The model under review builds one solid part; all positions refer to its coordinate system, in mm. Face numbers are marked on the shaded views. Round coordinates to 2 decimals unless told otherwise and drop trailing zeros. Write each loop counter-clockwise with the first axis right and the second up, starting at its lowest first coordinate (ties: lowest second). Pieces come first, ordered by that corner, then holes. Notation, with made-up numbers: (-10, 35) - (14, 35) arc R22 cw to (14, 52) - close; hole circle Ø5 at (49.25, 73.25). An arc over 180 degrees is marked (long way). One line per question, with ' | ' between items. Start each with the question number.
```python
from build123d import *

# Parameters (mm, degrees)
BOX202_W          = 16
BOX202_H          = 6
BOX202_DEPTH      = 2
BOX208_W          = 16
BOX208_H          = 6
BOX208_DEPTH      = 2
BOX206_W          = 16
BOX206_H          = 6
BOX206_DEPTH      = 2
BOX204_W          = 16
BOX204_H          = 6
BOX204_DEPTH      = 2
BOX198_W          = 16
BOX198_H          = 6
BOX198_DEPTH      = 2
BOX209_W          = 16
BOX209_H          = 6
BOX209_DEPTH      = 2
BOX205_W          = 16
BOX205_H          = 6
BOX205_DEPTH      = 2
BOX207_W          = 16
BOX207_H          = 6
BOX207_DEPTH      = 2
BOX200_W          = 16
BOX200_H          = 6
BOX200_DEPTH      = 2
BOX212_W          = 16
BOX212_H          = 6
BOX212_DEPTH      = 2
BOX211_W          = 16
BOX211_H          = 6
BOX211_DEPTH      = 2
BOX203_W          = 16
BOX203_H          = 6
BOX203_DEPTH      = 2
CYLINDER480_R     = 1.5
CYLINDER480_DEPTH = 50
CYLINDER467_R     = 1.5
CYLINDER467_DEPTH = 50
CYLINDER483_R     = 1.5
CYLINDER483_DEPTH = 50
CYLINDER486_R     = 1.5
CYLINDER486_DEPTH = 50
CYLINDER488_R     = 1.5
CYLINDER488_DEPTH = 50
CYLINDER482_R     = 1.5
CYLINDER482_DEPTH = 50
CYLINDER476_R     = 5
CYLINDER476_DEPTH = 100
CYLINDER475_R     = 5
CYLINDER475_DEPTH = 100
CYLINDER461_R     = 5
CYLINDER461_DEPTH = 100
CYLINDER477_R     = 5
CYLINDER477_DEPTH = 100
CYLINDER481_R     = 5
CYLINDER481_DEPTH = 100
CYLINDER478_R     = 5
CYLINDER478_DEPTH = 100
CYLINDER479_R     = 5
CYLINDER479_DEPTH = 100
CYLINDER474_R     = 5
CYLINDER474_DEPTH = 100
BOX201_W          = 10
BOX201_H          = 108
BOX201_DEPTH      = 20


with BuildPart() as krychle202:
    # Box202 → Box202 (new body)
    with BuildSketch(Plane(origin=(60, 2, 16), x_dir=(1, 0, 0), z_dir=(0, 0, 1))):
        with Locations((8, 3)):
            Rectangle(BOX202_W, BOX202_H)
    extrude(amount=BOX202_DEPTH)


with BuildPart() as krychle208:
    # Box208 → Box208 (new body)
    with BuildSketch(Plane(origin=(60, -21, 10), x_dir=(1, 0, 0), z_dir=(0, 0, 1))):
        with Locations((8, 3)):
            Rectangle(BOX208_W, BOX208_H)
    extrude(amount=BOX208_DEPTH)


with BuildPart() as krychle206:
    # Box206 → Box206 (new body)
    with BuildSketch(Plane(origin=(60, -21, 16), x_dir=(1, 0, 0), z_dir=(0, 0, 1))):
        with Locations((8, 3)):
            Rectangle(BOX206_W, BOX206_H)
    extrude(amount=BOX206_DEPTH)


with BuildPart() as krychle204:
    # Box204 → Box204 (new body)
    with BuildSketch(Plane(origin=(60, -41, 10), x_dir=(1, 0, 0), z_dir=(0, 0, 1))):
        with Locations((8, 3)):
            Rectangle(BOX204_W, BOX204_H)
    extrude(amount=BOX204_DEPTH)


with BuildPart() as krychle198:
    # Box198 → Box198 (new body)
    with BuildSketch(Plane(origin=(60, -41, 16), x_dir=(1, 0, 0), z_dir=(0, 0, 1))):
        with Locations((8, 3)):
            Rectangle(BOX198_W, BOX198_H)
    extrude(amount=BOX198_DEPTH)


with BuildPart() as krychle209:
    # Box209 → Box209 (new body)
    with BuildSketch(Plane(origin=(60, -51, 10), x_dir=(1, 0, 0), z_dir=(0, 0, 1))):
        with Locations((8, 3)):
            Rectangle(BOX209_W, BOX209_H)
    extrude(amount=BOX209_DEPTH)


with BuildPart() as krychle205:
    # Box205 → Box205 (new body)
    with BuildSketch(Plane(origin=(60, -51, 16), x_dir=(1, 0, 0), z_dir=(0, 0, 1))):
        with Locations((8, 3)):
            Rectangle(BOX205_W, BOX205_H)
    extrude(amount=BOX205_DEPTH)


with BuildPart() as krychle207:
    # Box207 → Box207 (new body)
    with BuildSketch(Plane(origin=(60, 30, 10), x_dir=(1, 0, 0), z_dir=(0, 0, 1))):
        with Locations((8, 3)):
            Rectangle(BOX207_W, BOX207_H)
    extrude(amount=BOX207_DEPTH)


with BuildPart() as krychle200:
    # Box200 → Box200 (new body)
    with BuildSketch(Plane(origin=(60, 46, 10), x_dir=(1, 0, 0), z_dir=(0, 0, 1))):
        with Locations((8, 3)):
            Rectangle(BOX200_W, BOX200_H)
    extrude(amount=BOX200_DEPTH)


with BuildPart() as krychle212:
    # Box212 → Box212 (new body)
    with BuildSketch(Plane(origin=(60, 30, 16), x_dir=(1, 0, 0), z_dir=(0, 0, 1))):
        with Locations((8, 3)):
            Rectangle(BOX212_W, BOX212_H)
    extrude(amount=BOX212_DEPTH)


with BuildPart() as krychle211:
    # Box211 → Box211 (new body)
    with BuildSketch(Plane(origin=(60, 46, 16), x_dir=(1, 0, 0), z_dir=(0, 0, 1))):
        with Locations((8, 3)):
            Rectangle(BOX211_W, BOX211_H)
    extrude(amount=BOX211_DEPTH)


with BuildPart() as compound592:
    # Box203 → Box203 (new body)
    with BuildSketch(Plane(origin=(60, 2, 10), x_dir=(1, 0, 0), z_dir=(0, 0, 1))):
        with Locations((8, 3)):
            Rectangle(BOX203_W, BOX203_H)
    extrude(amount=BOX203_DEPTH)

    # Compound592: union Krychle202, Krychle208, Krychle206, Krychle204, Krychle198, Krychle209, Krychle205, Krychle207, Krychle200, Krychle212, Krychle211
    add(krychle202.part)
    add(krychle208.part)
    add(krychle206.part)
    add(krychle204.part)
    add(krychle198.part)
    add(krychle209.part)
    add(krychle205.part)
    add(krychle207.part)
    add(krychle200.part)
    add(krychle212.part)
    add(krychle211.part)


with BuildPart() as compound592_1:
    # Compound592 placement: moved
    add(compound592.part.moved(Location((39, 24, 3))))


with BuildPart() as obj1:
    # Cylinder480 → Cylinder480 (new body)
    with BuildSketch(Plane(origin=(63, -18, -12), x_dir=(1, 0, 0), z_dir=(0, 0, 1))):
        Circle(CYLINDER480_R)
    extrude(amount=CYLINDER480_DEPTH)


with BuildPart() as obj2:
    # Cylinder467 → Cylinder467 (new body)
    with BuildSketch(Plane(origin=(63, -38, -12), x_dir=(1, 0, 0), z_dir=(0, 0, 1))):
        Circle(CYLINDER467_R)
    extrude(amount=CYLINDER467_DEPTH)


with BuildPart() as obj3:
    # Cylinder483 → Cylinder483 (new body)
    with BuildSketch(Plane(origin=(63, -48, -12), x_dir=(1, 0, 0), z_dir=(0, 0, 1))):
        Circle(CYLINDER483_R)
    extrude(amount=CYLINDER483_DEPTH)


with BuildPart() as obj4:
    # Cylinder486 → Cylinder486 (new body)
    with BuildSketch(Plane(origin=(63, 33, -12), x_dir=(1, 0, 0), z_dir=(0, 0, 1))):
        Circle(CYLINDER486_R)
    extrude(amount=CYLINDER486_DEPTH)


with BuildPart() as obj5:
    # Cylinder488 → Cylinder488 (new body)
    with BuildSketch(Plane(origin=(63, 49, -12), x_dir=(1, 0, 0), z_dir=(0, 0, 1))):
        Circle(CYLINDER488_R)
    extrude(amount=CYLINDER488_DEPTH)


with BuildPart() as compound593:
    # Cylinder482 → Cylinder482 (new body)
    with BuildSketch(Plane(origin=(63, 5, -12), x_dir=(1, 0, 0), z_dir=(0, 0, 1))):
        Circle(CYLINDER482_R)
    extrude(amount=CYLINDER482_DEPTH)

    # Compound593: union obj1, obj2, obj3, obj4, obj5
    add(obj1.part)
    add(obj2.part)
    add(obj3.part)
    add(obj4.part)
    add(obj5.part)


with BuildPart() as compound593_1:
    # Compound593 placement: moved
    add(compound593.part.moved(Location((39, 24, 0))))


with BuildPart() as obj6:
    # Cylinder476 → Cylinder476 (new body)
    with BuildSketch(Plane(origin=(24, -51, 25), x_dir=(0, 0, -1), z_dir=(1, 0, 0))):
        Circle(CYLINDER476_R)
    extrude(amount=CYLINDER476_DEPTH)


with BuildPart() as obj7:
    # Cylinder475 → Cylinder475 (new body)
    with BuildSketch(Plane(origin=(24, 36, 34), x_dir=(0, 0, -1), z_dir=(1, 0, 0))):
        Circle(CYLINDER475_R)
    extrude(amount=CYLINDER475_DEPTH)


with BuildPart() as obj8:
    # Cylinder461 → Cylinder461 (new body)
    with BuildSketch(Plane(origin=(24, -36, 34), x_dir=(0, 0, -1), z_dir=(1, 0, 0))):
        Circle(CYLINDER461_R)
    extrude(amount=CYLINDER461_DEPTH)


with BuildPart() as obj9:
    # Cylinder477 → Cylinder477 (new body)
    with BuildSketch(Plane(origin=(24, -23, -5), x_dir=(0, 0, -1), z_dir=(1, 0, 0))):
        Circle(CYLINDER477_R)
    extrude(amount=CYLINDER477_DEPTH)


with BuildPart() as obj10:
    # Cylinder481 → Cylinder481 (new body)
    with BuildSketch(Plane(origin=(24, 51, 7), x_dir=(0, 0, -1), z_dir=(1, 0, 0))):
        Circle(CYLINDER481_R)
    extrude(amount=CYLINDER481_DEPTH)


with BuildPart() as obj11:
    # Cylinder478 → Cylinder478 (new body)
    with BuildSketch(Plane(origin=(24, 23, -5), x_dir=(0, 0, -1), z_dir=(1, 0, 0))):
        Circle(CYLINDER478_R)
    extrude(amount=CYLINDER478_DEPTH)


with BuildPart() as obj12:
    # Cylinder479 → Cylinder479 (new body)
    with BuildSketch(Plane(origin=(24, -51, 7), x_dir=(0, 0, -1), z_dir=(1, 0, 0))):
        Circle(CYLINDER479_R)
    extrude(amount=CYLINDER479_DEPTH)


with BuildPart() as compound596:
    # Cylinder474 → Cylinder474 (new body)
    with BuildSketch(Plane(origin=(24, 51, 25), x_dir=(0, 0, -1), z_dir=(1, 0, 0))):
        Circle(CYLINDER474_R)
    extrude(amount=CYLINDER474_DEPTH)

    # Compound596: union obj6, obj7, obj8, obj9, obj10, obj11, obj12
    add(obj6.part)
    add(obj7.part)
    add(obj8.part)
    add(obj9.part)
    add(obj10.part)
    add(obj11.part)
    add(obj12.part)


with BuildPart() as compound596_1:
    # Compound596 placement: moved
    add(compound596.part.moved(Location((24, -6, 0))))


with BuildPart() as cut373:
    # Box201 → Box201 (new body)
    with BuildSketch(Plane(origin=(97, -29, 7), x_dir=(1, 0, 0), z_dir=(0, 0, 1))):
        with Locations((5, 54)):
            Rectangle(BOX201_W, BOX201_H)
    extrude(amount=BOX201_DEPTH)

    # Cut370: cut Compound596
    add(compound596_1.part, mode=Mode.SUBTRACT)

    # Cut372: cut Compound593
    add(compound593_1.part, mode=Mode.SUBTRACT)

    # Cut373: cut Compound592
    add(compound592_1.part, mode=Mode.SUBTRACT)


with BuildPart() as cut373_1:
    # Cut373 placement: moved
    add(cut373.part.moved(Location((8, 6, 0))))


solid = cut373_1.part
```
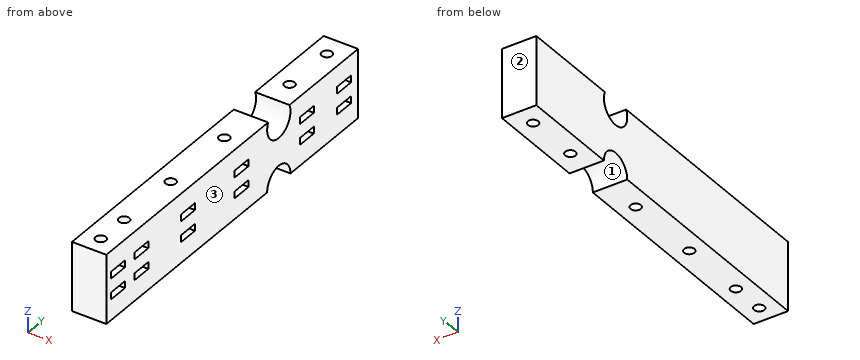
1. Add section C-C, the plane z = 25. Write out the cut boundary in (x, y), then the cut area to 3 significant figures.
2. Add section D-D, the plane x = 110. State how many separate pieces and enclosed holes the cut face has, then the cut area to 3 significant figures.
3. Wall thickness on line 1 along Z through (x, y) = (110.75, 37); line 2 along X through (y, z) = (79, 9.5); line 3 along X through (y, z) = (80, 12.75): over which ranges is each line inside the solid? List them lowest first. Write a range as [from, to].
4. Clearance check with flat-ended pins moving along their axes: P1, Ø2, axis at x = 112, y = 47.5, coming from the -Z side; P2, Ø0.6, axis at y = 62.5, z = 13.5, coming from the +X side; P3, Ø2.5, axis at x = 110, y = 79, coming from the +Z side. State where each tip first meets the part, or that it passes through.
5. Add section B-B, the plane y = 35. Write out the cut boundary in (x, z).
6. Add section A-A, the plane z = 9. Write out the cut boundary in (x, y), then the cut area to 3 significant figures.
7. The part is to be moulded in two halves that separate along Y. For the marked faces 1, 2 and 3, say which applies: pulls with the +Y half, pulls with the -Y half, needs draft (parallel to the pull), parting line crosses it, or undercut.
Geometry check:
1) outline: (105, -23) - (115, -23) - (115, 46) - (105, 46) - close; (105, 56) - (115, 56) - (115, 85) - (105, 85) - close; hole circle Ø3 at (110, -18); hole circle Ø3 at (110, -8); hole circle Ø3 at (110, 12); hole circle Ø3 at (110, 35); hole circle Ø3 at (110, 63); hole circle Ø3 at (110, 79) | area: 938 mm2
2) separate pieces: 7 | enclosed holes: 0 | area: 1,630 mm2
3) line 1: z = [7, 13], [15, 19], [21, 27] | line 2: x = [105, 108.5], [111.5, 115] | line 3: x = [105, 108.88], [111.12, 115]
4) P1: stops at z = 9.18 | P2: stops at x = 107 | P3: passes through
5) outline: (105, 7) - (108.5, 7) - (108.5, 13) - (107, 13) - (107, 15) - (108.5, 15) - (108.5, 19) - (107, 19) - (107, 21) - (108.5, 21) - (108.5, 27) - (105, 27) - close; (111.5, 7) - (115, 7) - (115, 13) - (111.5, 13) - close; (111.5, 15) - (115, 15) - (115, 19) - (111.5, 19) - close; (111.5, 21) - (115, 21) - (115, 27) - (111.5, 27) - close
6) outline: (105, -23) - (115, -23) - (115, 46.42) - (105, 46.42) - close; (105, 55.58) - (115, 55.58) - (115, 85) - (105, 85) - close; hole circle Ø3 at (110, -18); hole circle Ø3 at (110, -8); hole circle Ø3 at (110, 12); hole circle Ø3 at (110, 35); hole circle Ø3 at (110, 63); hole circle Ø3 at (110, 79) | area: 946 mm2
7) face 1: undercut | face 2: pulls with the +Y half | face 3: needs draft
